Design review of the part shown in the three views and the two pictorial views. Dimensions are in mm from the part's minimum x, y and z. A direction names the side the tool comes from. Coordinates: 2 decimals unless noted, no trailing zeros. Loops run counter-clockwise (first coordinate to the right, second up) from the corner with the lowest first, then second, coordinate; pieces in that order, holes last. Notation, with made-up numbers: (9, 55.25) -> (61, 55.25) arc R26 cw to (61, 75.25) -> close; hole circle Ø3 at (32, 27.25). An arc over 180 degrees is marked (long way). Use CSV: the item, a comma, the result in double quotes.
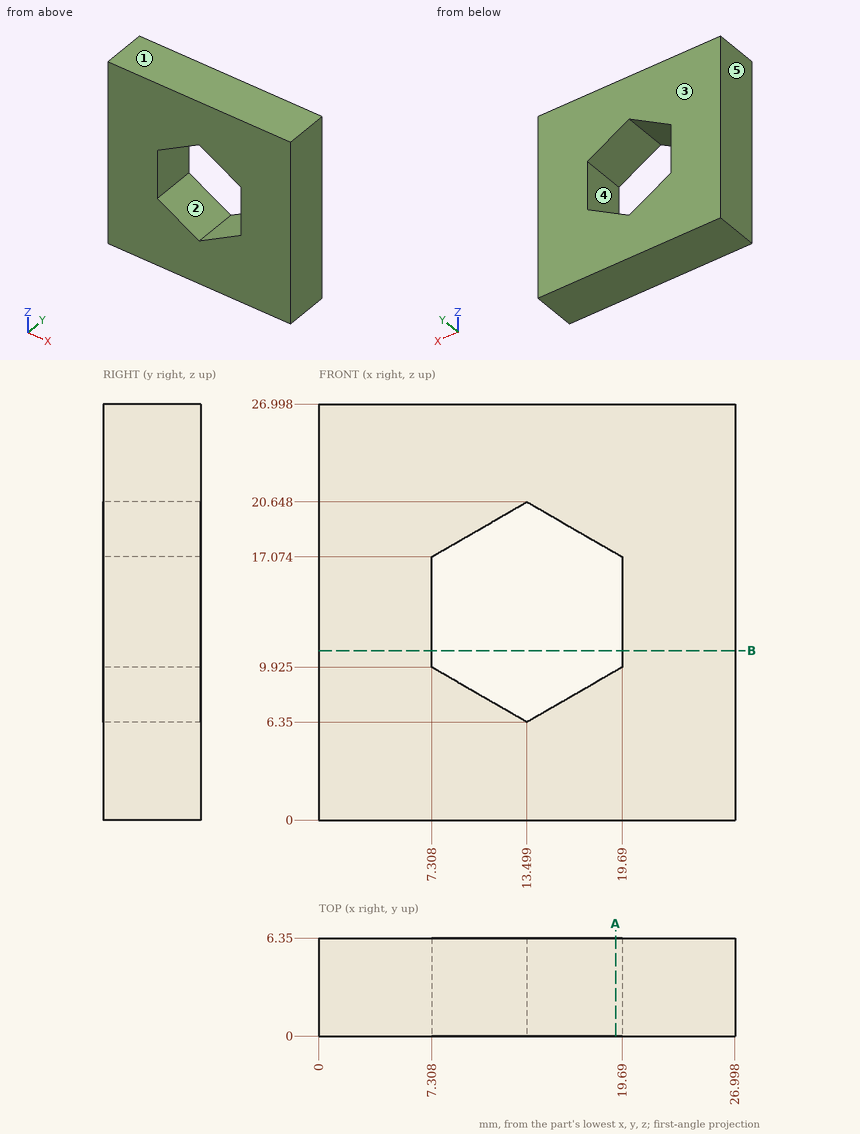
Item 1: To check wall thickness, follow line 1 along X through (y, z) = (0.75, 13.75); line 2 along Z through (x, y) = (14, 2.75); line 3 along Z through (x, y) = (9, 2). State the ranges of each line that lie inside material, in increasing order.
Checked values:
line 1,"0 to 7.31, 19.69 to 27"
line 2,"0 to 6.64, 20.36 to 27"
line 3,"0 to 8.95, 18.05 to 27"
Item 2: Add section A-A (x = 19.25). Give the boundary of the cut face in (y, z), then the cut area to 3 significant figures.
Checked values:
outline,"(0, 0) -> (6.35, 0) -> (6.35, 9.67) -> (0, 9.67) -> close; (0, 17.33) -> (6.35, 17.33) -> (6.35, 27) -> (0, 27) -> close"
area,"123 mm^2"
Item 3: Machinability: for the marked faces 1 and 2, which of the approach directions +Z, -Z, +X, -X, +Y, -Y give a long, thin tool a straight path to every point of the face, cutting with its end or side? Answer none if there is none.
Checked values:
face 1,"+Z, +X, -X, +Y, -Y"
face 2,"+Y, -Y"
Item 4: Add section B-B (z = 11). Give the boundary of the cut face in (x, y).
Checked values:
outline,"(0, 0) -> (7.31, 0) -> (7.31, 6.35) -> (0, 6.35) -> close; (19.69, 0) -> (27, 0) -> (27, 6.35) -> (19.69, 6.35) -> close"
Item 5: Clearance check with a flat-ended pin moving along its axis: pin 1 (3 mm diameter, centred on y = 4, z = 20.5, fed in from -X). State where the tip first meets the part, or that it passes through.
Checked values:
pin 1,"x = 0"
Item 6: Draft analysis for pull direction X (two halves, no side actions). For the marked faces 3, 4 and 5, state which applies: pulls with the +X half, pulls with the -X half, needs draft (parallel to the pull), parting line crosses it, or undercut.
Checked values:
face 3,"needs draft"
face 4,"undercut"
face 5,"pulls with the -X half"
